```python
from build123d import *

# Parameters (mm, degrees)
SKETCH_2_W               = 1.5
SKETCH_2_H               = 15.026279442
PATTERN_CIRCULAR_1_COUNT = 2
PATTERN_CIRCULAR_1_ANGLE = 120
CHAMFER_1_SIZE           = 0.2


with BuildPart() as part:
    # 草图1 → 旋转1 (revolve)
    with BuildSketch(Plane(origin=(0, 0, 0), x_dir=(0, 0, -1), z_dir=(1, 0, 0)), mode=Mode.PRIVATE) as revolve_1_sk:
        with BuildLine():
            Line((0, 4), (15, 4))
            Line((15, 4), (15, 5))
            Line((15, 5), (14.5, 5))
            Line((14.5, 5), (14.5, 11))
            Line((14.5, 11), (9.75, 11))
            Line((9.75, 11), (8.08660254, 8.118911087))
            ThreePointArc((8.08660254, 8.118911087), (8, 8.068911087), (7.91339746, 8.118911087))
            Line((7.91339746, 8.118911087), (6.25, 11))
            Line((6.25, 11), (4.75, 11))
            Line((4.75, 11), (3.08660254, 8.118911087))
            ThreePointArc((3.08660254, 8.118911087), (3, 8.068911087), (2.91339746, 8.118911087))
            Line((2.91339746, 8.118911087), (1.25, 11))
            Line((1.25, 11), (0, 11))
            Line((0, 11), (0, 4))
        make_face()
    revolve(revolve_1_sk.sketch.rotate(Axis((0, 0, 0), (0, 0, -1)), 90), axis=Axis((0, 0, 0), (0, 0, -1)))

    # 草图2 → M3 螺纹孔1 (revolve, cut)
    with BuildSketch(Plane(origin=(0, 0, -12.125), x_dir=(0, 0, -1), z_dir=(1, 0, 0))):
        with Locations((0.75, 7.513139721)):
            Rectangle(SKETCH_2_W, SKETCH_2_H)
    hole_wizard_m3_1 = revolve(axis=Axis((0, -6.35, -12.125), (0, 1, 0)), mode=Mode.SUBTRACT)

    # 阵列(圆周)1: M3 螺纹孔1 ×2 about axis
    pattern_circular_1_axis = Axis((0, 0, 0), (0, 0, 1))
    for i in range(1, PATTERN_CIRCULAR_1_COUNT):
        add(hole_wizard_m3_1.rotate(pattern_circular_1_axis, i * PATTERN_CIRCULAR_1_ANGLE / (PATTERN_CIRCULAR_1_COUNT - 1)), mode=Mode.SUBTRACT)

    # 倒角1
    chamfer_1_edges = [part.edges().sort_by_distance(p)[0] for p in [
        (-5, 0, -15),
        (-11, 0, 0),
        (-4, 0, 0),
        (-4, 0, -15),
    ]]
    chamfer(chamfer_1_edges, length=CHAMFER_1_SIZE)


solid = part.part
```
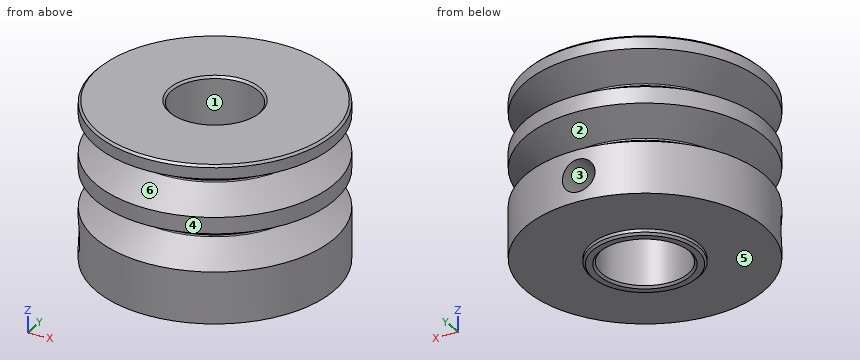
Here's how the part is built. I have some questions about the finished solid (model axes, mm). Face numbers are marked on the shaded views. A direction names the side the tool comes from. Round coordinates to 2 decimals unless told otherwise and drop trailing zeros. Write each loop counter-clockwise with the first axis right and the second up, starting at its lowest first coordinate (ties: lowest second). Pieces come first, ordered by that corner, then holes. Notation, with made-up numbers: M -9.5,-7 L -2.5,-7 A7 ccw -2.5,6 Z; hole C -4,3.25 d11. An arc over 180 degrees is marked long. Answer as CSV lines item,"result". Start each with the question number.
1. Suppose I cut it at B-B on x = 0. Count the separate pieces of the cut face and the enclosed holes in it, then the cut area to 3 significant figures.
2. On a 3-axis mill with a long thin cutter (end or side, diameter ignored), from which of +Z, -Z, +X, -X, +Y, -Y can I reach the whole of each face in a straight line? I mean the marked faces 1, 2 and 3. Say none if no direction works.
3. Thinking about a two-plate mould opening in Z: for the marked faces 4, 5 and 6, which applies, released by +Z, released by -Z, zero draft, split by the parting line, or undercut?
4. Suppose I cut it at A-A on z = -11.75. Write out the boundary of the cut face in (x, y), then the cut area to 3 significant figures.
5. I'm going to push flat-ended pins straight in: pin 1 Ø3 at (x, z) = (4, -4.5) entering from +Y; pin 2 Ø4 at (y, z) = (2, -7.5) entering from +X; pin 3 Ø5 at (y, z) = (4.5, -4) entering from -X; pin 4 Ø5 at (x, y) = (0, 0) entering from -Z. Where does each tip first touch, or does it pass through?
6. I need wall thicknesses on probe 1 along Y at (x, z) = (0, -10.5); probe 2 along Z at (x, y) = (4.25, -8.75); probe 3 along Z at (x, y) = (0, 9.25) (3 decimals). Which ranges of each line are inside material? Lowest first, please.
7. Suppose I cut it at D-D on z = -10.25. Write out the boundary of the cut face in (x, y), then the cut area to 3 significant figures.
Check result:
1,separate pieces,"3"
1,enclosed holes,"0"
1,area,"162 mm2"
2,face 1,"+Z, -Z"
2,face 2,"none"
2,face 3,"+Y"
3,face 4,"zero draft"
3,face 5,"released by -Z"
3,face 6,"undercut"
4,outline,"M -10.17,-4.19 L -3.95,-0.61 A4 cw -1.45,3.73 L -1.45,10.9 A11 ccw Z; M -8.72,-6.71 A11 ccw long 1.45,10.9 L 1.45,3.73 A4 cw long -2.5,-3.12 Z"
4,area,"289 mm2"
5,pin 1,"stops at y = 10.71"
5,pin 2,"stops at x = 10.99"
5,pin 3,"stops at x = -10.79"
5,pin 4,"passes through"
6,probe 1,"y = -11 to -4, 4 to 11"
6,probe 2,"z = -14.5 to -9.02, -6.98 to -4.02, -1.98 to 0"
6,probe 3,"z = -14.5 to -13.625, -10.625 to -8.74, -7.26 to -3.74, -2.26 to 0"
7,outline,"C 0,0 d22; hole C 0,0 d8"
7,area,"330 mm2"
